Autodesk Inventor part; units mm, degrees
ref_plane "YZ Plane" through (0, 0, 0) normal (1, 0, 0) x (0, 1, 0)
ref_plane "XZ Plane" through (0, 0, 0) normal (0, 1, 0) x (-1, 0, 0)
ref_plane "XY Plane" through (0, 0, 0) normal (0, 0, 1) x (1, 0, 0)
sketch "Sketch1" plane through (0, 0, 0) normal (0, 1, 0) x (-1, 0, 0)
  line L0 (-40, 75) -> (40, 75)
  line L1 (40, 75) -> (40, -75)
  line L2 (40, -75) -> (-40, -75)
  line L3 (-40, -75) -> (-40, 75)
  line L4 (-40, 75) -> (40, -75) construction
  line L5 (40, 75) -> (-40, -75) construction
  point P0 (0, 0)
  dimension "d0" = 80
  dimension "d1" = 150
extrude "Extrusion1" add sketch "Sketch1" along normal blind 3
sketch "Sketch2" plane through (0, 3, 0) normal (0, 1, 0) x (1, 0, 0)
  line L0 (-40, -75) -> (40, -75) construction
  line L1 (0, -75) -> (0, 75) construction
  line L2 (40, 75) -> (-40, 75) construction
  line L3 (40, -75) -> (40, 75) construction
  line L4 (40, 0) -> (-40, 0) construction
  line L5 (-40, 75) -> (-40, -75) construction
  line L6 (0, -75) -> (40, -75) construction
  line L7 (40, -75) -> (5, -75) construction
  line L8 (5, -75) -> (5, -35) construction
  line L9 (31.65, -69.3) -> (-21.65, -69.3) construction
  line L10 (-21.65, -69.3) -> (-21.65, -0.7) construction
  line L11 (-21.65, -0.7) -> (31.65, -0.7) construction
  line L12 (31.65, -0.7) -> (31.65, -69.3) construction
  line L13 (31.65, -69.3) -> (-21.65, -0.7) construction
  line L14 (-21.65, -69.3) -> (31.65, -0.7) construction
  line L15 (5, -69.3) -> (5, -55.3) construction
  line L16 (5, -55.3) -> (-21.65, -55.3) construction
  line L17 (5, -55.3) -> (31.65, -55.3) construction
  line L18 (-21.65, -54) -> (5, -54) construction
  line L19 (5, -54) -> (31.65, -54) construction
  line L20 (-21.65, -3.2) -> (5, -3.2) construction
  line L21 (5, -3.2) -> (31.65, -3.2) construction
  line L22 (31.65, -35) -> (29.15, -35) construction
  line L23 (29.15, -35) -> (29.15, -0.7) construction
  line L24 (29.15, -35) -> (29.15, -69.3) construction
  line L25 (24.05, -0.7) -> (24.05, -35) construction
  line L26 (24.05, -35) -> (24.05, -69.3) construction
  line L27 (-3.85, -0.7) -> (-3.85, -35) construction
  line L28 (-3.85, -35) -> (-3.85, -69.3) construction
  line L29 (-19.05, -0.7) -> (-19.05, -35) construction
  line L30 (-19.05, -35) -> (-19.05, -69.3) construction
  point P0 (0, 0)
  point P1 (-19.05, -54)
  point P2 (29.15, -55.3)
  point P3 (24.05, -3.2)
  point P4 (-3.85, -3.2)
  dimension "d4" = 35
  dimension "d5" = 40
  dimension "d6" = 53.3
  dimension "d7" = 68.6
  dimension "d8" = 14
  dimension "d9" = 1.3
  dimension "d10" = 50.8
  dimension "d11" = 2.5
  dimension "d12" = 5.1
  dimension "d13" = 27.9
  dimension "d14" = 15.2
hole "Hole1" at (-19.05, 3, 54) at (29.15, 3, 55.3) at (24.05, 3, 3.2) at (-3.85, 3, 3.2) direction (0, -1, 0) diameter 3.2 end through all
sketch "Sketch3" plane through (0, 3, 0) normal (0, 1, 0) x (1, 0, 0)
  line L0 (40, 75) -> (40, -75) construction
  line L1 (40, 75) -> (6.65, 75) construction
  line L2 (-40, 75) -> (40, 75) construction
  line L3 (6.65, 75) -> (6.65, 55) construction
  line L4 (-15.85, 16.5614) -> (29.15, 16.5614) construction
  line L5 (29.15, 16.5614) -> (29.15, 66.5614) construction
  line L6 (29.15, 66.5614) -> (-15.85, 66.5614) construction
  line L7 (-15.85, 66.5614) -> (-15.85, 16.5614) construction
  line L8 (-15.85, 16.5614) -> (29.15, 66.5614) construction
  line L9 (29.15, 16.5614) -> (-15.85, 66.5614) construction
  circle A0 centre (29.15, -55.3) radius 1.6 construction
  line L10 (29.15, -55.3) -> (40, -55.3) construction
  line L11 (29.15, -55.3) -> (29.15, 104.0464) construction
  point P0 (0, 0)
  point P1 (6.65, 41.5614)
  dimension "d22" = 33.35
  dimension "d23" = 20
  dimension "d24" = 45
  dimension "d25" = 50
  dimension "d26" = 10.85
  dimension "d27" = 10.85
hole "Hole2" at (-15.85, 3, -16.5614) at (-15.85, 3, -66.5614) at (29.15, 3, -16.5614) at (29.15, 3, -66.5614) direction (0, -1, 0) diameter 3.3 end through all
fillet "Fillet1" radius 4 4 edges at (40, 1.5, 75) (-40, 1.5, 75) (40, 1.5, -75) (-40, 1.5, -75)
sketch "Sketch4" plane through (0, 3, 0) normal (0, 1, 0) x (1, 0, 0)
  line L0 (-40, -75) -> (40, -75)
  line L1 (-40, 75) -> (-40, -75)
  line L2 (40, 75) -> (-40, 75)
  line L3 (40, -75) -> (40, 75)
  line L4 (36.5, 71.5) -> (-36.5, 71.5) construction
  line L5 (-36.5, 71.5) -> (-36.5, -71.5) construction
  line L6 (-36.5, -71.5) -> (36.5, -71.5) construction
  line L7 (36.5, -71.5) -> (36.5, 71.5) construction
  point P0 (0, 0)
  dimension "d36" = 3.5
hole "Hole3" at (-36.5, 3, 71.5) at (36.5, 3, 71.5) at (36.5, 3, -71.5) at (-36.5, 3, -71.5) direction (0, -1, 0) diameter 3.3 end through all
hole "Hole4" at (-30.1058, 3, -41.9761) direction (0, -1, 0) diameter 12 end through all
properties part number "plate"
Geometry check sheet. Reference: the model listing, model coordinates, mm. Round coordinates to 2 decimals unless told otherwise and drop trailing zeros. Order: outer loops, then holes, each group sorted by start corner. A loop starts at its lowest first (then second) coordinate and runs counter-clockwise, first axis right, second up. Notation, with made-up numbers: (78.25, 3.5) - (94.25, 3.5) arc R30 cw to (94.25, 33.5) - close; hole circle Ø8 at (-9.5, 59). An arc over 180 degrees is marked (long way). One line per question, with ' | ' between items. Start each with the question number.
(1) Depth check by flat-ended pin: pin 1 Ø2 at (x, z) = (36.5, -71.5) entering from -Y (3 decimals). Enter the tip coordinate at first touch or a pass-through.
(2) Sectioned sample at B-B on z = 3.2. Record the cut outline in (x, y).
(3) Release check for a two-part mould opening along Z. For faces 1 (the cylindrical face through (-38.859, 1.521, 73.797)), 2 (the flat face through (-1, 1, -75)), 3 (the cylindrical face through (-37.615, 1.479, 70.284)), 4 (the flat face through (1, 0, 1)) record: released by +Z, released by -Z, zero draft, split by the parting line, or undercut.
(4) Sectioned sample at C-C on x = -31.5. Record the cut outline in (y, z), and give its area (3 significant figures).
(5) Sectioned sample at D-D on y = 1.85. Count the separate pieces of the cut face and the enclosed holes in it, and give its area (3 significant figures).
(6) Sectioned sample at A-A on x = 29.15. Record the cut outline in (y, z), and give its area (3 significant figures).
(7) Thickness scan on L1, parallel to X at y = 1.05, z = -71.5; L2, parallel to Z at x = -36.5, y = 0.8; L3, parallel to Z at x = -15.85, y = 1.8. Record the ranges inside material, lowest first. Write a range as [from, to].
Conclusion:
1) pin 1: passes through
2) outline: (-40, 0) - (-5.45, 0) - (-5.45, 3) - (-40, 3) - close; (-2.25, 0) - (22.45, 0) - (22.45, 3) - (-2.25, 3) - close; (25.65, 0) - (40, 0) - (40, 3) - (25.65, 3) - close
3) face 1: released by +Z | face 2: released by -Z | face 3: undercut | face 4: zero draft
4) outline: (0, -75) - (3, -75) - (3, -47.81) - (0, -47.81) - close; (0, -36.14) - (3, -36.14) - (3, 75) - (0, 75) - close | area: 415 mm2
5) separate pieces: 1 | enclosed holes: 13 | area: 11,800 mm2
6) outline: (0, -75) - (3, -75) - (3, -68.21) - (0, -68.21) - close; (0, -64.91) - (3, -64.91) - (3, -18.21) - (0, -18.21) - close; (0, -14.91) - (3, -14.91) - (3, 53.7) - (0, 53.7) - close; (0, 56.9) - (3, 56.9) - (3, 75) - (0, 75) - close | area: 421 mm2
7) L1: x = [-39.97, -38.15], [-34.85, 34.85], [38.15, 39.97] | L2: z = [-74.97, -73.15], [-69.85, 69.85], [73.15, 74.97] | L3: z = [-75, -68.21], [-64.91, -18.21], [-14.91, 75]
